from build123d import *

# Parameters (mm, degrees)
EXTRUDE_1_DEPTH     = 3
SKETCH_2_R          = 1.5
CUT_EXTRUDE_1_DEPTH = 10
SKETCH_3_R          = 1.5
CUT_EXTRUDE_2_DEPTH = 10
SKETCH_4_R          = 1.5
CUT_EXTRUDE_3_DEPTH = 3


with BuildPart() as part:
    # 草图1 → 凸台-拉伸1 (new body)
    with BuildSketch(Plane(origin=(0, 0, 0), x_dir=(1, 0, 0), z_dir=(0, 1, 0))):
        with BuildLine():
            Line((-65.342005187, 0), (65.342005187, 0))
            ThreePointArc((65.342005187, 0), (72.407706971, -2.923570229), (75.341993678, -9.984828338))
            add(Edge.make_bspline(
                [(75.341993678, -9.984828338), (75.362629964, -23.586675416), (71.657087991, -49.894617792), (60.538848208, -73.890924153), (53.072976878, -85.431659706)],
                knots=[0.101765917, 0.101765917, 0.101765917, 0.101765917, 0.521592529, 0.943927148, 0.943927148, 0.943927148, 0.943927148], degree=3))
            ThreePointArc((53.072976878, -85.431659706), (49.456022644, -88.783979652), (44.676723378, -90))
            Line((44.676723378, -90), (-44.676723378, -90))
            ThreePointArc((-44.676723378, -90), (-49.456022644, -88.783979652), (-53.072976878, -85.431659706))
            add(Edge.make_bspline(
                [(-75.341993678, -9.984828338), (-75.362629964, -23.586675416), (-71.657087991, -49.894617792), (-60.538848208, -73.890924153), (-53.072976878, -85.431659706)],
                knots=[0.101765917, 0.101765917, 0.101765917, 0.101765917, 0.521592529, 0.943927148, 0.943927148, 0.943927148, 0.943927148], degree=3))
            ThreePointArc((-75.341993678, -9.984828338), (-72.407706971, -2.923570229), (-65.342005187, 0))
        make_face()
    extrude(amount=EXTRUDE_1_DEPTH)

    # 草图2 → 切除-拉伸1 (cut)
    with BuildSketch(Plane(origin=(0, 3, 0), x_dir=(1, 0, 0), z_dir=(0, 1, 0))):
        with Locations(Location((-65.342005187, -10, 0), (0, 0, 270))):
            Circle(SKETCH_2_R)
        with Locations(Location((-46.986453842, -83.497243756, 0), (0, 0, 270))):
            Circle(SKETCH_2_R)
        with Locations(Location((46.986453842, -83.497243756, 0), (0, 0, 90))):
            Circle(SKETCH_2_R)
        with Locations(Location((65.342005187, -10, 0), (0, 0, 90))):
            Circle(SKETCH_2_R)
    extrude(amount=-CUT_EXTRUDE_1_DEPTH, mode=Mode.SUBTRACT)

    # 草图3 → 切除-拉伸2 (cut)
    with BuildSketch(Plane(origin=(0, 3, 0), x_dir=(1, 0, 0), z_dir=(0, 1, 0))):
        with Locations(Location((-28.387774848, -7.340263553, 0), (0, 0, 270))):
            Circle(SKETCH_3_R)
        with Locations(Location((27.718646552, -7.340263553, 0), (0, 0, 270))):
            Circle(SKETCH_3_R)
        with Locations(Location((19.695499635, -77.462033559, 0), (0, 0, 270))):
            Circle(SKETCH_3_R)
        with Locations(Location((-20.384564295, -77.521997213, 0), (0, 0, 270))):
            Circle(SKETCH_3_R)
    extrude(amount=-CUT_EXTRUDE_2_DEPTH, mode=Mode.SUBTRACT)

    # 草图4 → 切除-拉伸3 (cut)
    with BuildSketch(Plane(origin=(0, 3, 0), x_dir=(1, 0, 0), z_dir=(0, 1, 0))):
        with Locations(Location((-58.033655971, -65.458214846, 0), (0, 0, 270))):
            Circle(SKETCH_4_R)
        with Locations(Location((58.033655971, -65.458214846, 0), (0, 0, 90))):
            Circle(SKETCH_4_R)
    extrude(amount=-CUT_EXTRUDE_3_DEPTH, mode=Mode.SUBTRACT)


solid = part.part
Design review of the part built by this model. Coordinates are the model's own, in mm. Coordinates: 2 decimals unless noted, no trailing zeros. Use one line per item in the form item = value.
(1) Draft analysis for pull direction Z (two halves, no side actions). For faces 1 (the face through (-49.39, 1.48, 88.82)), 2 (the face through (72.33, 1.479, 2.846)), 3 (the face through (-27.374, 1.521, 6.235)), state which applies: pulls with the +Z half, pulls with the -Z half, needs draft (parallel to the pull), parting line crosses it, or undercut.
Return value:
face_1 = pulls with the +Z half
face_2 = pulls with the -Z half
face_3 = undercut
(2) Clearance check with flat-ended pins moving along their axes: P1, Ø2.5, axis at x = 58.03, z = 65.46, coming from the +Y side; P2, Ø1.5, axis at y = 1.5, z = 43.5, coming from the -X side. State where each tip first meets the part, or that it passes through.
Return value:
P1 = through
P2 = -71.56
(3) Consider section A-A (y = 1.4). Give the number of separate pieces and of enclosed holes in the cut face, and give its area (3 significant figures).
Return value:
separate_pieces = 1
enclosed_holes = 10
area = 12,200 mm2
(4) For line 1 along X through (y, z) = (0.8, 10); line 2 along X through (y, z) = (1.4, 12.5); line 3 along Z through (x, y) = (64, 1.4), list the stretches that pass through material, from the lowest coordinate up. Write a range as from..to.
Return value:
line_1 = -75.34..-66.84, -63.84..63.84, 66.84..75.34
line_2 = -75.32..75.32
line_3 = 0..9.33, 10.67..65.2
